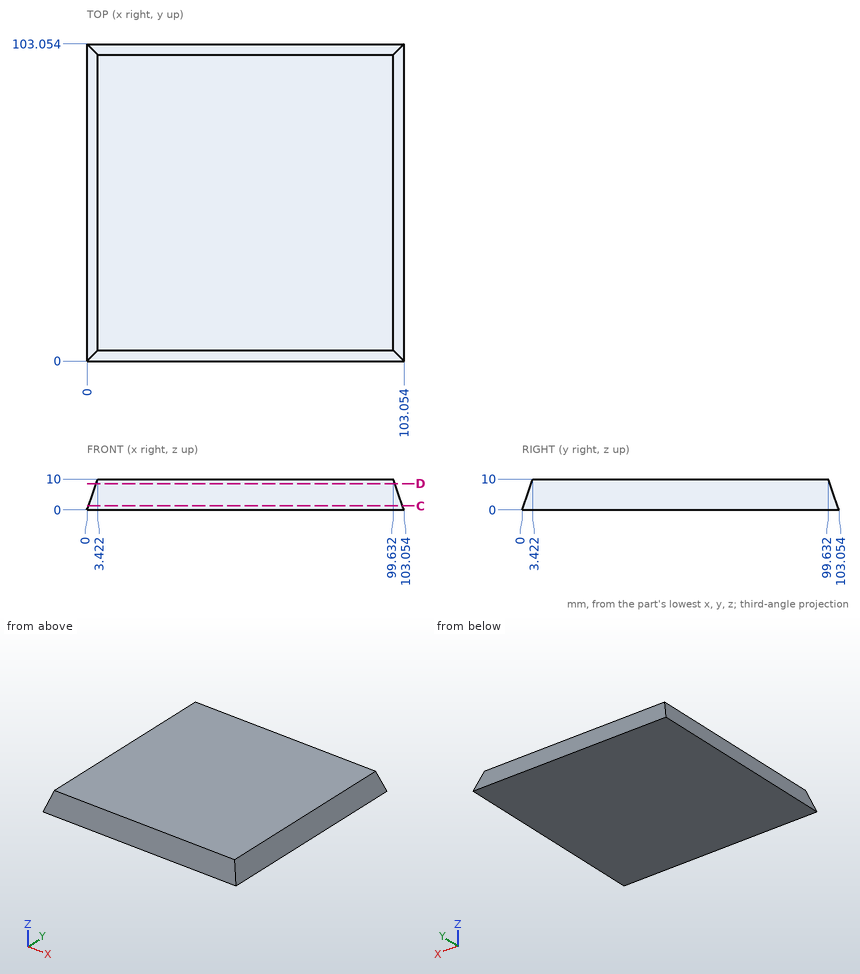
Input: dimensioned drawing with shaded views. Units: mm. Origin: part minimum x, y, z. Give positions to 0.01 mm unless a question says otherwise; leave off trailing zeros. Order: outer loops, then holes, each group sorted by start corner. A loop starts at its lowest first (then second) coordinate and runs counter-clockwise, first axis right, second up.
(1) Section query C-C (z = 1.25). Return the cut outline in (x, y), plus the area to 3 significant figures.
(2) Section query D-D (z = 8.5). Return the cut outline in (x, y) (1 decimal), plus the area to 4 significant figures.
(3) Contact query for flat-ended pins moving along their axis: P1, Ø2, axis at x = 18.5, z = 4, coming from the +Y side; P2, Ø1, axis at x = 27.5, z = 4, coming from the -Y side; P3, Ø2, axis at x = 52, z = 2, coming from the +Y side. Output: stop coordinate, or through.
(4) Material intervals for line 1 along Y through (x, z) = (86, 4.5) (1 decimal); line 2 along Y through (x, z) = (99, 3); line 3 along X through (y, z) = (36.5, 1.5), sorted ascending.
Outcome:
1. outline: (0.43, 0.43) - (102.63, 0.43) - (102.63, 102.63) - (0.43, 102.63) - close
1. area: 10,400 mm2
2. outline: (2.9, 2.9) - (100.1, 2.9) - (100.1, 100.1) - (2.9, 100.1) - close
2. area: 9,455 mm2
3. P1: stops at y = 102.03
3. P2: stops at y = 1.2
3. P3: stops at y = 102.71
4. line 1: y = 1.5 to 101.5
4. line 2: y = 1.03 to 102.03
4. line 3: x = 0.51 to 102.54
